Can you work these out from the model? Positions are in its coordinate system, mm. A direction names the side the tool comes from. Round coordinates to 2 decimals unless told otherwise and drop trailing zeros. Loops run counter-clockwise (first coordinate to the right, second up) from the corner with the lowest first, then second, coordinate; pieces in that order, holes last. Notation, with made-up numbers: (-22.75, 49.5) -> (35.25, 49.5) arc R31 cw to (35.25, 73.5) -> close; hole circle Ø7 at (36.25, 81.25). An arc over 180 degrees is marked (long way). Write item = value, one per line.
from build123d import *

# Parameters (mm, degrees)
SKETCH4_R           = 63.5
SKETCH4_R_2         = 50.8
BOSS_EXTRUDE4_DEPTH = 12.7
SKETCH1_R           = 50.8
SKETCH1_R_2         = 3.175
BOSS_EXTRUDE5_DEPTH = 2.54


with BuildPart() as part:
    # Sketch4 → Boss-Extrude4 (new body)
    with BuildSketch(Plane.XY):
        Circle(SKETCH4_R)
        Circle(SKETCH4_R_2, mode=Mode.SUBTRACT)
    extrude(amount=BOSS_EXTRUDE4_DEPTH)

    # Sketch1 → Boss-Extrude5 (add)
    with BuildSketch(Plane.XY):
        Circle(SKETCH1_R)
        with Locations((-44.45, 0)):
            Circle(SKETCH1_R_2, mode=Mode.SUBTRACT)
        with Locations((-42.475211217, 13.101867503)):
            Circle(SKETCH1_R_2, mode=Mode.SUBTRACT)
        with Locations((-36.726313518, 25.039576581)):
            Circle(SKETCH1_R_2, mode=Mode.SUBTRACT)
        with Locations((-27.714121693, 34.752409396)):
            Circle(SKETCH1_R_2, mode=Mode.SUBTRACT)
        with Locations((-16.239408533, 41.377338127)):
            Circle(SKETCH1_R_2, mode=Mode.SUBTRACT)
        with Locations((-3.32175266, 44.325708785)):
            Circle(SKETCH1_R_2, mode=Mode.SUBTRACT)
        with Locations((9.891055514, 43.335545696)):
            Circle(SKETCH1_R_2, mode=Mode.SUBTRACT)
        with Locations((22.225, 38.494829198)):
            Circle(SKETCH1_R_2, mode=Mode.SUBTRACT)
        with Locations((32.584155703, 30.233678194)):
            Circle(SKETCH1_R_2, mode=Mode.SUBTRACT)
        with Locations((40.048066178, 19.286132204)):
            Circle(SKETCH1_R_2, mode=Mode.SUBTRACT)
        with Locations((43.953530226, 6.624928732)):
            Circle(SKETCH1_R_2, mode=Mode.SUBTRACT)
        with Locations((43.953530226, -6.624928732)):
            Circle(SKETCH1_R_2, mode=Mode.SUBTRACT)
        with Locations((40.048066178, -19.286132204)):
            Circle(SKETCH1_R_2, mode=Mode.SUBTRACT)
        with Locations((32.584155703, -30.233678194)):
            Circle(SKETCH1_R_2, mode=Mode.SUBTRACT)
        with Locations((22.225, -38.494829198)):
            Circle(SKETCH1_R_2, mode=Mode.SUBTRACT)
        with Locations((9.891055514, -43.335545696)):
            Circle(SKETCH1_R_2, mode=Mode.SUBTRACT)
        with Locations((-3.32175266, -44.325708785)):
            Circle(SKETCH1_R_2, mode=Mode.SUBTRACT)
        with Locations((-16.239408533, -41.377338127)):
            Circle(SKETCH1_R_2, mode=Mode.SUBTRACT)
        with Locations((-27.714121693, -34.752409396)):
            Circle(SKETCH1_R_2, mode=Mode.SUBTRACT)
        with Locations((-36.726313518, -25.039576581)):
            Circle(SKETCH1_R_2, mode=Mode.SUBTRACT)
        with Locations((-42.475211217, -13.101867503)):
            Circle(SKETCH1_R_2, mode=Mode.SUBTRACT)
    extrude(amount=BOSS_EXTRUDE5_DEPTH)


solid = part.part
1. Suppose I cut it at B-B, the plane x = -43.5. List the corners of the cut face in (y, z) for me.
Entries:
outline = (-46.26, 0) -> (-16.11, 0) -> (-16.11, 2.54) -> (-26.24, 2.54) -> (-26.24, 12.7) -> (-46.26, 12.7) -> close; (-10.1, 0) -> (-3.03, 0) -> (-3.03, 2.54) -> (-10.1, 2.54) -> close; (3.03, 0) -> (10.1, 0) -> (10.1, 2.54) -> (3.03, 2.54) -> close; (16.11, 0) -> (46.26, 0) -> (46.26, 12.7) -> (26.24, 12.7) -> (26.24, 2.54) -> (16.11, 2.54) -> close
2. Suppose I cut it at C-C, the plane z = 6.75. List the corners of the cut face in (x, y) for me, and give its area (3 significant figures).
Entries:
outline = circle Ø127 at (0, 0); hole circle Ø101.6 at (0, 0)
area = 4,560 mm²
3. For faces 4 (the cylindrical face through (11.6, 46.01, 1.25)), 5 (the cylindrical face through (-11.012, -49.592, 7.549)), which set-ups out of +Z, -Z, +X, -X, +Y, -Y let a thin tool reach every point of the face, with its end or its side?
Entries:
face_4 = +Z, -Z
face_5 = +Z
4. Suppose I cut it at A-A, the plane y = 0. List the corners of the cut face in (x, z) for me (3 decimals), and give its area (3 significant figures).
Entries:
outline = (-63.5, 0) -> (-47.625, 0) -> (-47.625, 2.54) -> (-50.8, 2.54) -> (-50.8, 12.7) -> (-63.5, 12.7) -> close; (-41.275, 0) -> (63.5, 0) -> (63.5, 12.7) -> (50.8, 12.7) -> (50.8, 2.54) -> (-41.275, 2.54) -> close
area = 565 mm²
5. I need wall thicknesses on line 1 (X direction, y = 33, z = 0.5); line 2 (Y direction, x = 0, z = 7); line 3 (Y direction, x = -16, z = 2). Which ranges of each line are inside material? Lowest first, please. Write a range as [from, to].
Entries:
line_1 = [-54.25, -30.36], [-25.07, 31.03], [34.14, 54.25]
line_2 = [-63.5, -50.8], [50.8, 63.5]
line_3 = [-61.45, -44.54], [-38.21, 38.21], [44.54, 61.45]
6. We'd pull the mould along X, two halves only. Please class faces 1 (the cylindrical face through (-14.533, 44.055, 1.252)), 2 (the flat face through (-29, 43, 12.7)), 3 (the flat face through (-1, 1, 2.54)): released by +X, released by -X, zero draft, split by the parting line, or undercut.
Entries:
face_1 = undercut
face_2 = zero draft
face_3 = undercut
7. Suppose I cut it at D-D, the plane x = -2.5. List the corners of the cut face in (y, z) for me.
Entries:
outline = (-63.45, 0) -> (-47.39, 0) -> (-47.39, 2.54) -> (-50.74, 2.54) -> (-50.74, 12.7) -> (-63.45, 12.7) -> close; (-41.26, 0) -> (41.26, 0) -> (41.26, 2.54) -> (-41.26, 2.54) -> close; (47.39, 0) -> (63.45, 0) -> (63.45, 12.7) -> (50.74, 12.7) -> (50.74, 2.54) -> (47.39, 2.54) -> close
8. I'm going to push flat-ended pins straight in: pin 1 (8 mm diameter, centred on x = -35, y = 21.5, fed in from -Z); pin 2 (6 mm diameter, centred on x = 9, z = 4.5, fed in from -Y); pin 3 (8.5 mm diameter, centred on x = -16.24, y = 41.38, fed in from +Z); pin 4 (1.5 mm diameter, centred on x = 10, z = 3.5, fed in from -Y). Where does each tip first touch, or does it pass through?
Entries:
pin_1 = 0
pin_2 = -63.22
pin_3 = 2.54
pin_4 = -62.82
